Can you work these out from the drawing? Everything is in mm from the part's minimum corner. Give positions to 0.01 mm unless a question says otherwise; leave off trailing zeros. Order: outer loops, then holes, each group sorted by start corner. A loop starts at its lowest first (then second) coordinate and runs counter-clockwise, first axis right, second up. Notation, with made-up numbers: (72, -14.75) - (94, -14.75) arc R23 cw to (94, 2.25) - close; hole circle Ø6 at (65.25, -40). An arc over 180 degrees is marked (long way). Write each question's results on one line, items separated by ' | '. Start each with the question number.
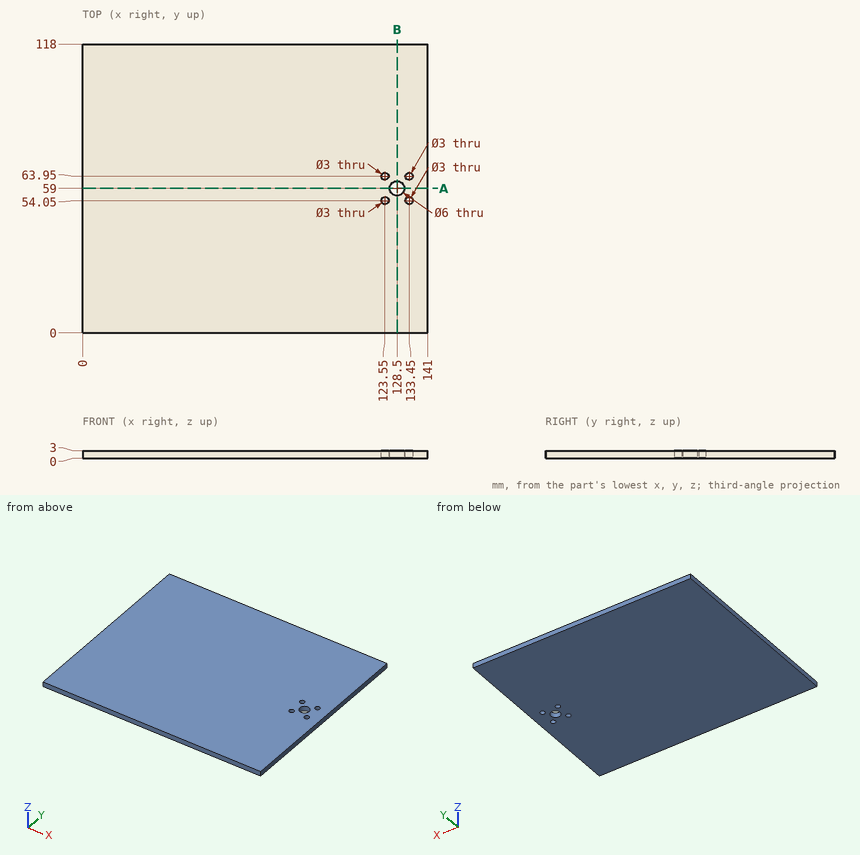
Q1. If we section it at A-A (y = 59): Please give me the cut outline in (x, z), plus the area to 3 significant figures.
Q2. Will this pin go through, and if not, where does the flat tip stop? P1, Ø1.8, axis at x = 133.45, y = 54.05, coming from the -Z side.
Q3. If we section it at B-B (x = 128.5): Please give me the cut outline in (y, z).
Q4. If I drill on probe 1 along X at (y, z) = (64, 2.15); probe 2 along Y at (x, z) = (133.5, 2.4); probe 3 along Y at (x, z) = (128.5, 0.9), over which ranges is the centre line in solid material (lowest first)? Write a range as from..to.
Findings below:
1) outline: (0, 0) - (125.5, 0) - (125.5, 3) - (0, 3) - close; (131.5, 0) - (141, 0) - (141, 3) - (131.5, 3) - close | area: 405 mm2
2) P1: passes through
3) outline: (0, 0) - (56, 0) - (56, 3) - (0, 3) - close; (62, 0) - (118, 0) - (118, 3) - (62, 3) - close
4) probe 1: x = 0..122.05, 125.05..131.95, 134.95..141 | probe 2: y = 0..52.55, 55.55..62.45, 65.45..118 | probe 3: y = 0..56, 62..118
